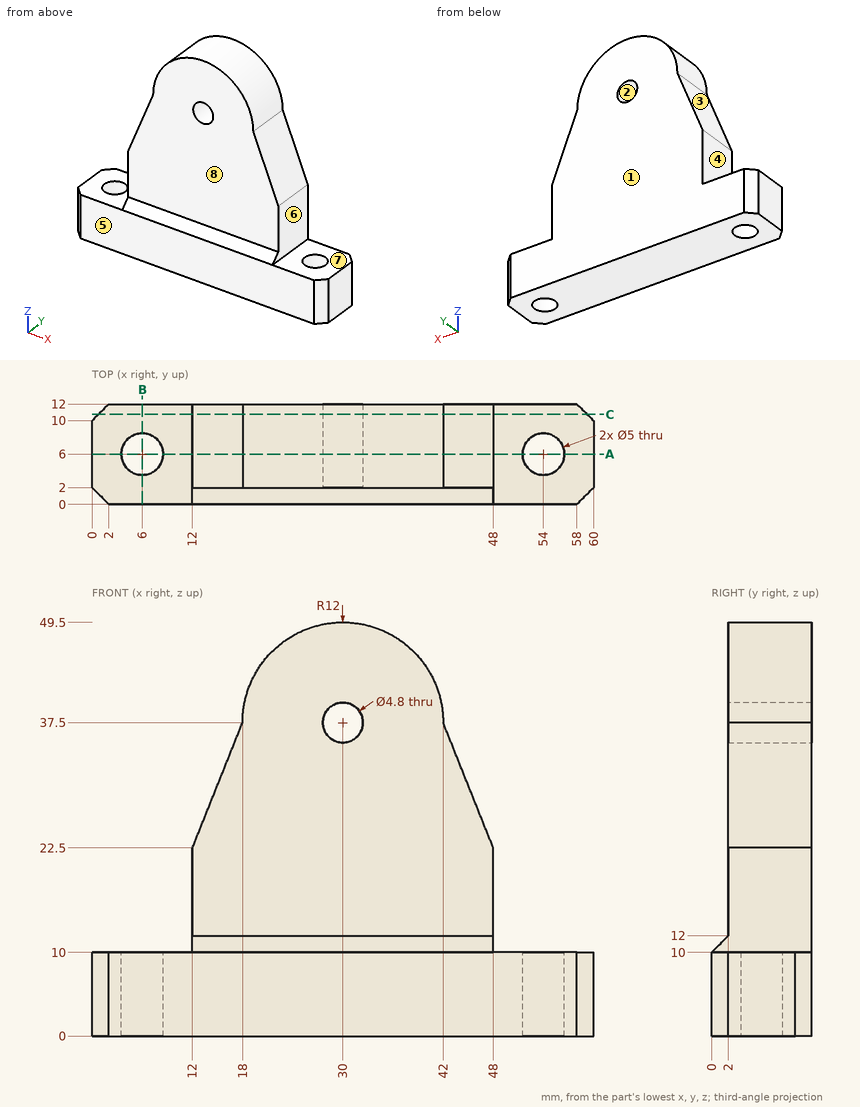
Geometry: see drawing. Coordinates: mm, zero at the bounding-box minimum. A direction names the side the tool comes from. Give positions to 0.01 mm unless a question says otherwise; leave off trailing zeros. Order: outer loops, then holes, each group sorted by start corner. A loop starts at its lowest first (then second) coordinate and runs counter-clockwise, first axis right, second up. Notation, with made-up numbers: (9.25, -14.75) - (56.25, -14.75) arc R19 cw to (56.25, -4.75) - close; hole circle Ø4 at (56.25, 3). An arc over 180 degrees is marked (long way). Use CSV: the item, a comma, the result in double quotes.
1. Access query for the marked faces 4, 5, 6, 7 and 8. Directions: +Z, -Z, +X, -X, +Y, -Y. A direction counts if a zero-diameter tool reaches every point of the face in a straight line with its end or side. Return the directions, or none.
Answers below:
face 4,"+Z, -X, +Y, -Y"
face 5,"+Z, -Z, +X, -X, -Y"
face 6,"+Z, +X, +Y, -Y"
face 7,"+Z, +X, +Y, -Y"
face 8,"+Z, +X, -X, -Y"
2. Contact query for flat-ended pins moving along their axis: pin 1 (3 mm diameter, centred on y = 10, z = 35.5, fed in from +X); pin 2 (6 mm diameter, centred on x = 16, y = 5, fed in from +Z) (1 decimal); pin 3 (1.5 mm diameter, centred on y = 9.5, z = 13.5, fed in from +X); pin 4 (4 mm diameter, centred on x = 6, y = 6, fed in from -Z). Output: stop coordinate, or through.
Answers below:
pin 1,"x = 43.4"
pin 2,"z = 42.3"
pin 3,"x = 48"
pin 4,"through"
3. Mould query, pull axis X, two halves, no side actions, for the marked faces 1, 2 and 3. Classes: +X half, -X half, draft (parallel to the pull), parting line (faces both ways), or undercut.
Answers below:
face 1,"draft"
face 2,"undercut"
face 3,"-X half"
4. Material intervals for line 1 along X through (y, z) = (6, 7.25); line 2 along Z through (x, y) = (30, 5.5); line 3 along X through (y, z) = (9.25, 18), sorted ascending. Write a range as from..to.
Answers below:
line 1,"0..3.5, 8.5..51.5, 56.5..60"
line 2,"0..35.1, 39.9..49.5"
line 3,"12..48"
5. Section query A-A (y = 6). Output: boundary loops of the cut face in (x, z), plus the area to 3 significant figures.
Answers below:
outline,"(0, 0) - (3.5, 0) - (3.5, 10) - (0, 10) - close; (8.5, 0) - (51.5, 0) - (51.5, 10) - (48, 10) - (48, 22.5) - (42, 37.5) arc R12 ccw to (18, 37.5) - (12, 22.5) - (12, 10) - (8.5, 10) - close; (56.5, 0) - (60, 0) - (60, 10) - (56.5, 10) - close; hole circle Ø4.8 at (30, 37.5)"
area,"1,610 mm2"
6. Section query C-C (y = 10.75). Output: boundary loops of the cut face in (x, z).
Answers below:
outline,"(0.75, 0) - (59.25, 0) - (59.25, 10) - (48, 10) - (48, 22.5) - (42, 37.5) arc R12 ccw to (18, 37.5) - (12, 22.5) - (12, 10) - (0.75, 10) - close; hole circle Ø4.8 at (30, 37.5)"
7. Section query B-B (x = 6). Output: boundary loops of the cut face in (y, z).
Answers below:
outline,"(0, 0) - (3.5, 0) - (3.5, 10) - (0, 10) - close; (8.5, 0) - (12, 0) - (12, 10) - (8.5, 10) - close"
